Geometry: see drawing. Coordinates: mm, zero at the bounding-box minimum. Round coordinates to 2 decimals unless told otherwise and drop trailing zeros. Loops run counter-clockwise (first coordinate to the right, second up) from the corner with the lowest first, then second, coordinate; pieces in that order, holes last. Notation, with made-up numbers: (84, 46.5) -> (119, 46.5) arc R13 cw to (119, 67.5) -> close; hole circle Ø8 at (32, 59.25). An arc over 180 degrees is marked (long way). Answer in a Markdown table with one row per item.
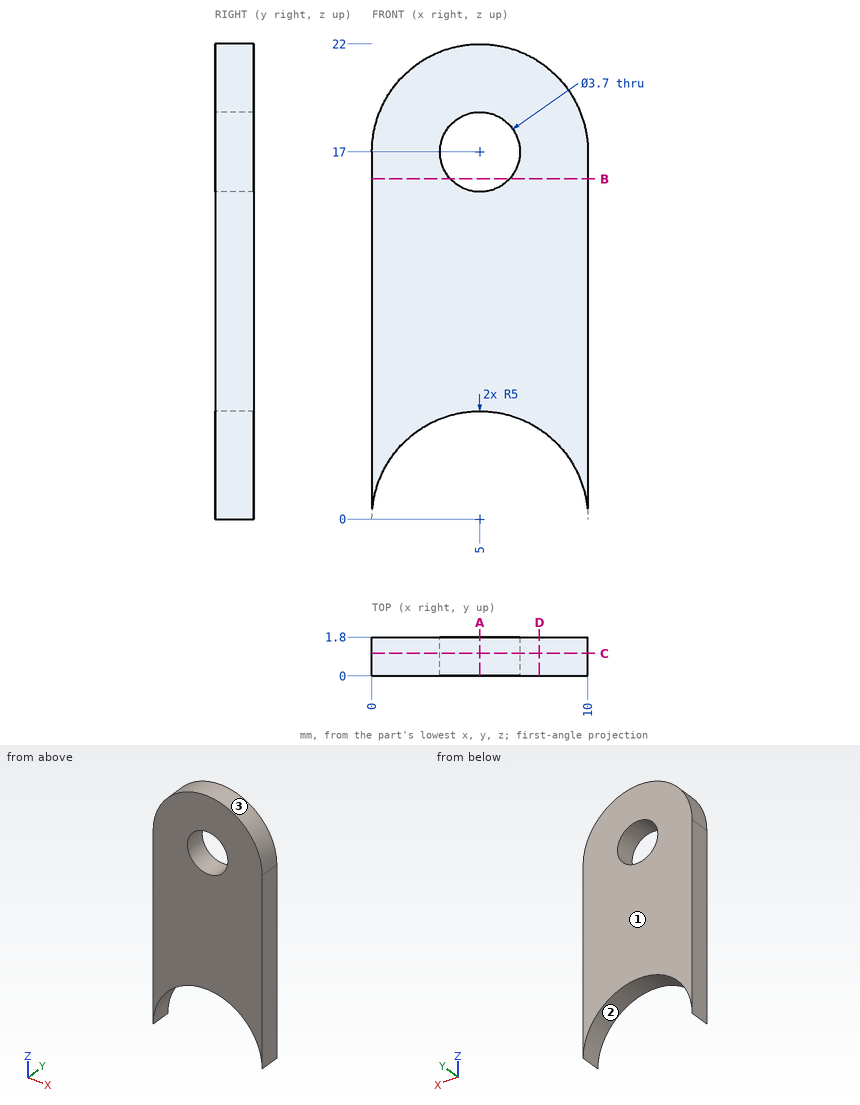
Item 1: Mould query, pull axis X, two halves, no side actions, for the marked faces 1, 2 and 3. Classes: released by +X, released by -X, zero draft, split by the parting line, or undercut.
Ans:
| item | result |
|---|---|
| face 1 | zero draft |
| face 2 | undercut |
| face 3 | split by the parting line |
Item 2: Section query C-C, the plane y = 1.05. Output: boundary loops of the cut face in (x, z).
Ans:
| item | result |
|---|---|
| outline | (0, 0) arc R5 cw to (10, 0) -> (10, 17) arc R5 ccw to (0, 17) -> close; hole circle Ø3.7 at (5, 17) |
Item 3: Section query B-B, the plane z = 15.75. Output: boundary loops of the cut face in (x, y).
Ans:
| item | result |
|---|---|
| outline | (0, 0) -> (3.64, 0) -> (3.64, 1.8) -> (0, 1.8) -> close; (6.36, 0) -> (10, 0) -> (10, 1.8) -> (6.36, 1.8) -> close |
Item 4: Section query A-A, the plane x = 5. Output: boundary loops of the cut face in (y, z), and give its area (3 significant figures).
Ans:
| item | result |
|---|---|
| outline | (0, 5) -> (1.8, 5) -> (1.8, 15.15) -> (0, 15.15) -> close; (0, 18.85) -> (1.8, 18.85) -> (1.8, 22) -> (0, 22) -> close |
| area | 23.9 mm2 |
Item 5: Ray query, L1, parallel to Z at x = 5, y = 0.95; L2, parallel to Z at x = 4, y = 1.45; L3, parallel to X at y = 1.55, z = 19.5. Return the intervals inside material, ascending.
Ans:
| item | result |
|---|---|
| L1 | 5 to 15.15, 18.85 to 22 |
| L2 | 4.9 to 15.44, 18.56 to 21.9 |
| L3 | 0.67 to 9.33 |
Item 6: Section query D-D, the plane x = 7.75. Output: boundary loops of the cut face in (y, z), and give its area (3 significant figures).
Ans:
| item | result |
|---|---|
| outline | (0, 4.18) -> (1.8, 4.18) -> (1.8, 21.18) -> (0, 21.18) -> close |
| area | 30.6 mm2 |
